Design review of the part shown in the three views and the two pictorial views. Dimensions are in mm from the part's minimum x, y and z. Round coordinates to 2 decimals unless told otherwise and drop trailing zeros. Loops run counter-clockwise (first coordinate to the right, second up) from the corner with the lowest first, then second, coordinate; pieces in that order, holes last. Notation, with made-up numbers: M 68.25,81.25 L 73.25,81.25 A25 ccw 73.25,105.25 Z; hole C 29.25,4.25 d9. An arc over 180 degrees is marked long. One line per question, with ' | ' between items. Start each with the question number.
1) For pin 1 Ø4 at (x, y) = (32.5, 18) entering from -Z, flat-tipped, find the tip position at first contact; note if it passes through.
2) We need section A-A (y = 12.5). Give the boundary of the cut face in (x, z) (3 decimals).
3) We need section D-D (y = 5.5). Give the boundary of the cut face in (x, z) (3 decimals).
4) We need section B-B (z = 2.4). Give the boundary of the cut face in (x, y).
5) For probe 1 along X at (y, z) = (12.5, 1.55); probe 2 along Y at (x, z) = (11, 2.5); probe 3 along Y at (x, z) = (8, 2.4), list the stretches that pass through material, from the lowest coordinate up. Write a range as from..to.
6) Mouldability with a two-part tool opening along Z and no side actions: class the marked faces 1 and 2 as pulls with the +Z half, pulls with the -Z half, needs draft (parallel to the pull), parting line crosses it, or undercut.
7) We need section C-C (x = 79). Give the boundary of the cut face in (y, z) (3 decimals), and give its area (3 significant figures).
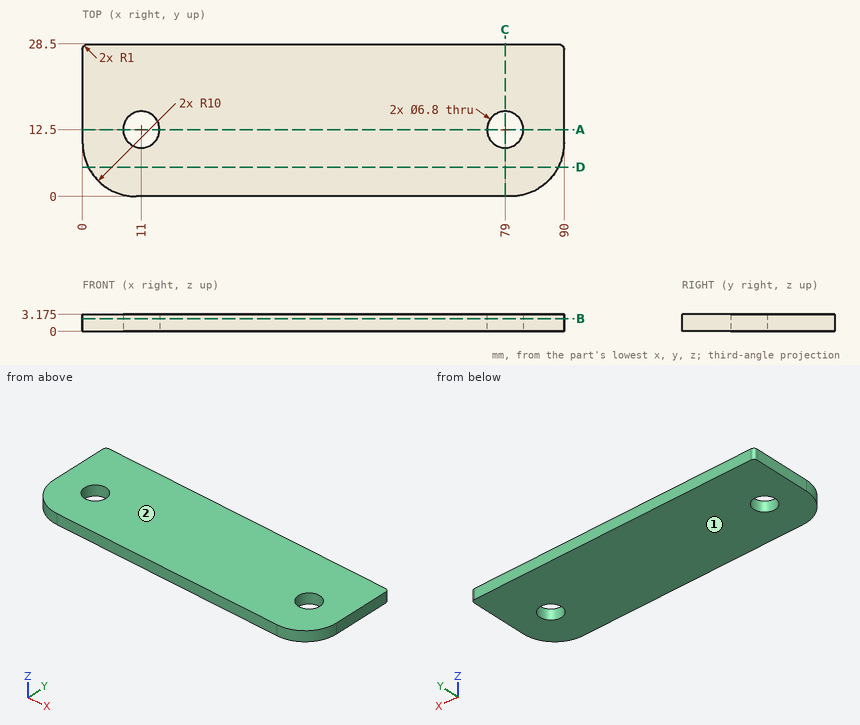
Answers below:
1) pin 1: z = 0
2) outline: M 0,0 L 7.6,0 L 7.6,3.175 L 0,3.175 Z; M 14.4,0 L 75.6,0 L 75.6,3.175 L 14.4,3.175 Z; M 82.4,0 L 90,0 L 90,3.175 L 82.4,3.175 Z
3) outline: M 1.07,0 L 88.93,0 L 88.93,3.175 L 1.07,3.175 Z
4) outline: M 0,10 A10 ccw 10,0 L 80,0 A10 ccw 90,10 L 90,27.5 A1 ccw 89,28.5 L 1,28.5 A1 ccw 0,27.5 Z; hole C 11,12.5 d6.8; hole C 79,12.5 d6.8
5) probe 1: 0..7.6, 14.4..75.6, 82.4..90 | probe 2: 0..9.1, 15.9..28.5 | probe 3: 0.2..10.9, 14.1..28.5
6) face 1: pulls with the -Z half | face 2: pulls with the +Z half
7) outline: M 0,0 L 9.1,0 L 9.1,3.175 L 0,3.175 Z; M 15.9,0 L 28.5,0 L 28.5,3.175 L 15.9,3.175 Z | area: 68.9 mm^2
